Here's how the part is built. I have some questions about the finished solid (model axes, mm). A direction names the side the tool comes from. Coordinates: 2 decimals unless noted, no trailing zeros. Write each loop counter-clockwise with the first axis right and the second up, starting at its lowest first coordinate (ties: lowest second). Pieces come first, ordered by that corner, then holes.
Autodesk Inventor part; units mm, degrees
ref_plane "YZ Plane" through (0, 0, 0) normal (1, 0, 0) x (0, 1, 0)
ref_plane "XZ Plane" through (0, 0, 0) normal (0, 1, 0) x (-1, 0, 0)
ref_plane "XY Plane" through (0, 0, 0) normal (0, 0, 1) x (1, 0, 0)
sketch "Sketch1" plane through (0, 0, 0) normal (1, 0, 0) x (0, 1, 0)
  line L0 (0, 90) -> (330, 90)
  line L1 (330, 90) -> (330, -90)
  line L2 (330, -90) -> (0, -90)
  line L3 (0, -90) -> (0, 90)
  line L4 (0, 0) -> (345.997, 0) construction
  dimension "d0" = 330
  dimension "d1" = 180
extrude "Extrusion1" add sketch "Sketch1" along normal blind 120
sketch "Sketch2" plane through (120, 0, 0) normal (1, 0, 0) x (0, 0, -1)
  line L0 (-5.1081, 224.8212) -> (8.9019, 224.8212) construction
  line L1 (8.9019, 224.8212) -> (8.9019, 216.6905) construction
  line L2 (8.9019, 216.6905) -> (-5.1081, 216.6905) construction
  line L3 (-5.1081, 216.6905) -> (-5.1081, 224.8212) construction
  point P0 (0, 0)
hole "Hole1" at (0, 280, 0) direction (1, 0, 0) diameter 25.4 depth 25.4
properties part number "RFI_power_filter"
1) We'd pull the mould along Y, two halves only. Please class faces 1 (the face through (59, 0, -1)), 2 (the face through (59, 330, 1)), 3 (the face through (59, 167, -90)), 4 (the face through (12.878, 267.408, -1.653)): pulls with the +Y half, pulls with the -Y half, needs draft (parallel to the pull), parting line crosses it, or undercut.
Values follow:
face 1: pulls with the -Y half
face 2: pulls with the +Y half
face 3: needs draft
face 4: undercut
2) Imagine slicing it at B-B on z = 0. Please give me the cut outline in (x, y).
Values follow:
outline: (0, 0) - (120, 0) - (120, 330) - (0, 330) - (0, 292.7) - (25.4, 292.7) - (25.4, 267.3) - (0, 267.3) - close
3) Will this pin go through, and if not, where does the flat tip stop? pin 1 (7.5 mm diameter, centred on y = 281, z = 4, fed in from -X).
Values follow:
pin 1: stops at x = 25.4
4) I need wall thicknesses on probe 1 along Y at (x, z) = (9, 0); probe 2 along Z at (x, y) = (19, 280). Which ranges of each line are inside material? Lowest first, please.
Values follow:
probe 1: y = 0 to 267.3, 292.7 to 330
probe 2: z = -90 to -12.7, 12.7 to 90
5) On a 3-axis mill with a long thin cutter (end or side, diameter ignored), from which of +Z, -Z, +X, -X, +Y, -Y can I reach the whole of each face in a straight line? I mean faces 5 (the face through (25.4, 280, 0)), 6 (the face through (120, 163, 1)). Say none if no direction works.
Values follow:
face 5: -X
face 6: +Z, -Z, +X, +Y, -Y
6) Imagine slicing it at A-A on y = 280. Please give me the cut outline in (x, z), then the cut area to 3 significant figures.
Values follow:
outline: (0, -90) - (120, -90) - (120, 90) - (0, 90) - (0, 12.7) - (25.4, 12.7) - (25.4, -12.7) - (0, -12.7) - close
area: 21,000 mm2
